```python
from build123d import *

# Parameters (mm, degrees)
SKETCH1_W            = 54.5
SKETCH1_H            = 146
BOSS_EXTRUDE1_DEPTH  = 1.75
SKETCH2_R            = 3.5
SKETCH2_R_2          = 3.795961701
SKETCH2_R_3          = 8
CUT_EXTRUDE1_DEPTH   = 78.939880677
M3_CLEARANCE_HOLE1_D = 3.6
FILLET1_R            = 5


with BuildPart() as part:
    # Sketch1 → Boss-Extrude1 (new body)
    with BuildSketch(Plane(origin=(0, 0, 0), x_dir=(1, 0, 0), z_dir=(0, 1, 0))):
        Rectangle(SKETCH1_W, SKETCH1_H)
    extrude(amount=BOSS_EXTRUDE1_DEPTH)

    # Sketch2 → Cut-Extrude1 (cut, through all)
    with BuildSketch(Plane(origin=(0, 1.75, 0), x_dir=(1, 0, 0), z_dir=(0, 1, 0))):
        with Locations(Location((-19.25, 57, 0), (0, 0, 270))):
            Circle(SKETCH2_R)
        with Locations(Location((-19.25, 0, 0), (0, 0, 270))):
            Circle(SKETCH2_R_2)
        with Locations(Location((-19.25, -57, 0), (0, 0, 90))):
            Circle(SKETCH2_R)
        with Locations(Location((19.25, -57, 0), (0, 0, 270))):
            Circle(SKETCH2_R)
        with Locations(Location((19.25, 0, 0), (0, 0, 90))):
            Circle(SKETCH2_R_2)
        with Locations(Location((19.25, 57, 0), (0, 0, 90))):
            Circle(SKETCH2_R)
        with Locations(Location((0, 0, 0), (0, 0, 270))):
            Circle(SKETCH2_R_3)
        with BuildLine():
            Line((-11.737972568, 9.475230868), (-23.68137085, 21.41862915))
            ThreePointArc((-23.68137085, 21.41862915), (-23.68137085, 23.68137085), (-21.41862915, 23.68137085))
            Line((-21.41862915, 23.68137085), (-9.475230868, 11.737972568))
            ThreePointArc((-9.475230868, 11.737972568), (-9.475230868, 9.475230868), (-11.737972568, 9.475230868))
        make_face()
        with BuildLine():
            Line((11.737972568, 9.475230868), (23.68137085, 21.41862915))
            ThreePointArc((23.68137085, 21.41862915), (23.68137085, 23.68137085), (21.41862915, 23.68137085))
            Line((21.41862915, 23.68137085), (9.475230868, 11.737972568))
            ThreePointArc((9.475230868, 11.737972568), (9.475230868, 9.475230868), (11.737972568, 9.475230868))
        make_face()
        with BuildLine():
            Line((-11.737972568, -9.475230868), (-23.68137085, -21.41862915))
            ThreePointArc((-23.68137085, -21.41862915), (-23.68137085, -23.68137085), (-21.41862915, -23.68137085))
            Line((-21.41862915, -23.68137085), (-9.475230868, -11.737972568))
            ThreePointArc((-9.475230868, -11.737972568), (-9.475230868, -9.475230868), (-11.737972568, -9.475230868))
        make_face()
        with BuildLine():
            Line((11.737972568, -9.475230868), (23.68137085, -21.41862915))
            ThreePointArc((23.68137085, -21.41862915), (23.68137085, -23.68137085), (21.41862915, -23.68137085))
            Line((21.41862915, -23.68137085), (9.475230868, -11.737972568))
            ThreePointArc((9.475230868, -11.737972568), (9.475230868, -9.475230868), (11.737972568, -9.475230868))
        make_face()
        with BuildLine():
            Line((-9.357792216, 68.20993346), (-6.161205405, 68.20993346))
            ThreePointArc((-6.161205405, 68.20993346), (-3.661205405, 65.70993346), (-6.161205405, 63.20993346))
            Line((-6.161205405, 63.20993346), (-9.357792216, 63.20993346))
            ThreePointArc((-9.357792216, 63.20993346), (-11.857792216, 65.70993346), (-9.357792216, 68.20993346))
        make_face()
        with BuildLine():
            Line((-9.357792216, 58.20993346), (-6.161205405, 58.20993346))
            ThreePointArc((-6.161205405, 58.20993346), (-3.661205405, 55.70993346), (-6.161205405, 53.20993346))
            Line((-6.161205405, 53.20993346), (-9.357792216, 53.20993346))
            ThreePointArc((-9.357792216, 53.20993346), (-11.857792216, 55.70993346), (-9.357792216, 58.20993346))
        make_face()
        with BuildLine():
            Line((9.357792216, 58.20993346), (6.161205405, 58.20993346))
            ThreePointArc((6.161205405, 58.20993346), (3.661205405, 55.70993346), (6.161205405, 53.20993346))
            Line((6.161205405, 53.20993346), (9.357792216, 53.20993346))
            ThreePointArc((9.357792216, 53.20993346), (11.857792216, 55.70993346), (9.357792216, 58.20993346))
        make_face()
        with BuildLine():
            Line((-9.357792216, 48.20993346), (-6.161205405, 48.20993346))
            ThreePointArc((-6.161205405, 48.20993346), (-3.661205405, 45.70993346), (-6.161205405, 43.20993346))
            Line((-6.161205405, 43.20993346), (-9.357792216, 43.20993346))
            ThreePointArc((-9.357792216, 43.20993346), (-11.857792216, 45.70993346), (-9.357792216, 48.20993346))
        make_face()
        with BuildLine():
            Line((9.357792216, 48.20993346), (6.161205405, 48.20993346))
            ThreePointArc((6.161205405, 48.20993346), (3.661205405, 45.70993346), (6.161205405, 43.20993346))
            Line((6.161205405, 43.20993346), (9.357792216, 43.20993346))
            ThreePointArc((9.357792216, 43.20993346), (11.857792216, 45.70993346), (9.357792216, 48.20993346))
        make_face()
        with BuildLine():
            Line((-9.357792216, 38.20993346), (-6.161205405, 38.20993346))
            ThreePointArc((-6.161205405, 38.20993346), (-3.661205405, 35.70993346), (-6.161205405, 33.20993346))
            Line((-6.161205405, 33.20993346), (-9.357792216, 33.20993346))
            ThreePointArc((-9.357792216, 33.20993346), (-11.857792216, 35.70993346), (-9.357792216, 38.20993346))
        make_face()
        with BuildLine():
            Line((9.357792216, 68.20993346), (6.161205405, 68.20993346))
            ThreePointArc((6.161205405, 68.20993346), (3.661205405, 65.70993346), (6.161205405, 63.20993346))
            Line((6.161205405, 63.20993346), (9.357792216, 63.20993346))
            ThreePointArc((9.357792216, 63.20993346), (11.857792216, 65.70993346), (9.357792216, 68.20993346))
        make_face()
        with BuildLine():
            Line((9.357792216, 38.20993346), (6.161205405, 38.20993346))
            ThreePointArc((6.161205405, 38.20993346), (3.661205405, 35.70993346), (6.161205405, 33.20993346))
            Line((6.161205405, 33.20993346), (9.357792216, 33.20993346))
            ThreePointArc((9.357792216, 33.20993346), (11.857792216, 35.70993346), (9.357792216, 38.20993346))
        make_face()
        with BuildLine():
            Line((-9.357792216, 28.20993346), (-6.161205405, 28.20993346))
            ThreePointArc((-6.161205405, 28.20993346), (-3.661205405, 25.70993346), (-6.161205405, 23.20993346))
            Line((-6.161205405, 23.20993346), (-9.357792216, 23.20993346))
            ThreePointArc((-9.357792216, 23.20993346), (-11.857792216, 25.70993346), (-9.357792216, 28.20993346))
        make_face()
        with BuildLine():
            Line((9.357792216, 28.20993346), (6.161205405, 28.20993346))
            ThreePointArc((6.161205405, 28.20993346), (3.661205405, 25.70993346), (6.161205405, 23.20993346))
            Line((6.161205405, 23.20993346), (9.357792216, 23.20993346))
            ThreePointArc((9.357792216, 23.20993346), (11.857792216, 25.70993346), (9.357792216, 28.20993346))
        make_face()
        with BuildLine():
            Line((-9.357792216, -68.20993346), (-6.161205405, -68.20993346))
            ThreePointArc((-6.161205405, -68.20993346), (-3.661205405, -65.70993346), (-6.161205405, -63.20993346))
            Line((-6.161205405, -63.20993346), (-9.357792216, -63.20993346))
            ThreePointArc((-9.357792216, -63.20993346), (-11.857792216, -65.70993346), (-9.357792216, -68.20993346))
        make_face()
        with BuildLine():
            Line((-9.357792216, -58.20993346), (-6.161205405, -58.20993346))
            ThreePointArc((-6.161205405, -58.20993346), (-3.661205405, -55.70993346), (-6.161205405, -53.20993346))
            Line((-6.161205405, -53.20993346), (-9.357792216, -53.20993346))
            ThreePointArc((-9.357792216, -53.20993346), (-11.857792216, -55.70993346), (-9.357792216, -58.20993346))
        make_face()
        with BuildLine():
            Line((9.357792216, -58.20993346), (6.161205405, -58.20993346))
            ThreePointArc((6.161205405, -58.20993346), (3.661205405, -55.70993346), (6.161205405, -53.20993346))
            Line((6.161205405, -53.20993346), (9.357792216, -53.20993346))
            ThreePointArc((9.357792216, -53.20993346), (11.857792216, -55.70993346), (9.357792216, -58.20993346))
        make_face()
        with BuildLine():
            Line((-9.357792216, -48.20993346), (-6.161205405, -48.20993346))
            ThreePointArc((-6.161205405, -48.20993346), (-3.661205405, -45.70993346), (-6.161205405, -43.20993346))
            Line((-6.161205405, -43.20993346), (-9.357792216, -43.20993346))
            ThreePointArc((-9.357792216, -43.20993346), (-11.857792216, -45.70993346), (-9.357792216, -48.20993346))
        make_face()
        with BuildLine():
            Line((9.357792216, -48.20993346), (6.161205405, -48.20993346))
            ThreePointArc((6.161205405, -48.20993346), (3.661205405, -45.70993346), (6.161205405, -43.20993346))
            Line((6.161205405, -43.20993346), (9.357792216, -43.20993346))
            ThreePointArc((9.357792216, -43.20993346), (11.857792216, -45.70993346), (9.357792216, -48.20993346))
        make_face()
        with BuildLine():
            Line((-9.357792216, -38.20993346), (-6.161205405, -38.20993346))
            ThreePointArc((-6.161205405, -38.20993346), (-3.661205405, -35.70993346), (-6.161205405, -33.20993346))
            Line((-6.161205405, -33.20993346), (-9.357792216, -33.20993346))
            ThreePointArc((-9.357792216, -33.20993346), (-11.857792216, -35.70993346), (-9.357792216, -38.20993346))
        make_face()
        with BuildLine():
            Line((9.357792216, -68.20993346), (6.161205405, -68.20993346))
            ThreePointArc((6.161205405, -68.20993346), (3.661205405, -65.70993346), (6.161205405, -63.20993346))
            Line((6.161205405, -63.20993346), (9.357792216, -63.20993346))
            ThreePointArc((9.357792216, -63.20993346), (11.857792216, -65.70993346), (9.357792216, -68.20993346))
        make_face()
        with BuildLine():
            Line((9.357792216, -38.20993346), (6.161205405, -38.20993346))
            ThreePointArc((6.161205405, -38.20993346), (3.661205405, -35.70993346), (6.161205405, -33.20993346))
            Line((6.161205405, -33.20993346), (9.357792216, -33.20993346))
            ThreePointArc((9.357792216, -33.20993346), (11.857792216, -35.70993346), (9.357792216, -38.20993346))
        make_face()
        with BuildLine():
            Line((-9.357792216, -28.20993346), (-6.161205405, -28.20993346))
            ThreePointArc((-6.161205405, -28.20993346), (-3.661205405, -25.70993346), (-6.161205405, -23.20993346))
            Line((-6.161205405, -23.20993346), (-9.357792216, -23.20993346))
            ThreePointArc((-9.357792216, -23.20993346), (-11.857792216, -25.70993346), (-9.357792216, -28.20993346))
        make_face()
        with BuildLine():
            Line((9.357792216, -28.20993346), (6.161205405, -28.20993346))
            ThreePointArc((6.161205405, -28.20993346), (3.661205405, -25.70993346), (6.161205405, -23.20993346))
            Line((6.161205405, -23.20993346), (9.357792216, -23.20993346))
            ThreePointArc((9.357792216, -23.20993346), (11.857792216, -25.70993346), (9.357792216, -28.20993346))
        make_face()
    extrude(amount=-CUT_EXTRUDE1_DEPTH, mode=Mode.SUBTRACT)

    # M3 Clearance Hole1 (through all)
    with Locations(Plane(origin=(0, 1.75, 0), x_dir=(1, 0, 0), z_dir=(0, 1, 0))):
        with Locations((-21.25, 67), (21.25, -67), (-21.25, -67), (-21.25, 31), (21.25, 67), (21.25, 31), (21.25, -31), (-21.25, -31), (-15.25, -7.65)):
            Hole(M3_CLEARANCE_HOLE1_D / 2)

    # Fillet1
    fillet1_edges = [part.edges().sort_by_distance(p)[0] for p in [
        (27.25, 0.875, 73),
        (-27.25, 0.875, 73),
        (-27.25, 0.875, -73),
        (27.25, 0.875, -73),
    ]]
    fillet(fillet1_edges, radius=FILLET1_R)


solid = part.part
```
Could you check a few things on this model? Use its own coordinates, in mm. Coordinates: 2 decimals unless noted, no trailing zeros. Order: outer loops, then holes, each group sorted by start corner. A loop starts at its lowest first (then second) coordinate and runs counter-clockwise, first axis right, second up. Notation, with made-up numbers: M 81,-7.75 L 135,-7.75 A26 cw 135,11.25 Z; hole C -6,84.5 d10. An arc over 180 degrees is marked long. Use one line per item in the form item = value. Start each with the question number.
1. Suppose I cut it at B-B on x = 0. Write out the boundary of the cut face in (y, z), then the cut area to 4 significant figures.
2. Suppose I cut it at D-D on y = 1.25. Count the separate pieces of the cut face and the enclosed holes in it, then the cut area to 3 significant figures.
3. Suppose I cut it at C-C on z = 0. Write out the boundary of the cut face in (x, y), then the cut area to 3 significant figures.
4. Suppose I cut it at A-A on z = -31. Write out the boundary of the cut face in (x, y).
5. We'd pull the mould along Z, two halves only. Please class faces 1 (the cylindrical face through (-25.82, 0.89, 71.5)), 2 (the cylindrical face through (3.66, 0.89, -25.76)): +Z half, -Z half, draft (parallel to the pull), parting line (faces both ways), or undercut.
6. Please list where these lines run through material, in increasing order: line 1 (X direction, y = 0.8, z = 0); line 2 (X direction, y = 0.25, z = 59); line 3 (X direction, y = 0.4, z = -31).
Geometry says:
q1.outline = M 0,-73 L 1.75,-73 L 1.75,-8 L 0,-8 Z; M 0,8 L 1.75,8 L 1.75,73 L 0,73 Z
q1.area = 227.5 mm^2
q2.separate_pieces = 1
q2.enclosed_holes = 40
q2.area = 6,440 mm^2
q3.outline = M -27.25,0 L -23.05,0 L -23.05,1.75 L -27.25,1.75 Z; M -15.45,0 L -8,0 L -8,1.75 L -15.45,1.75 Z; M 8,0 L 15.45,0 L 15.45,1.75 L 8,1.75 Z; M 23.05,0 L 27.25,0 L 27.25,1.75 L 23.05,1.75 Z
q3.area = 40.8 mm^2
q4.outline = M -27.25,0 L -23.05,0 L -23.05,1.75 L -27.25,1.75 Z; M -19.45,0 L 19.45,0 L 19.45,1.75 L -19.45,1.75 Z; M 23.05,0 L 27.25,0 L 27.25,1.75 L 23.05,1.75 Z
q5.face_1 = +Z half
q5.face_2 = undercut
q6.line_1 = -27.25 to -23.05, -15.45 to -8, 8 to 15.45, 23.05 to 27.25
q6.line_2 = -27.25 to -22.12, -16.38 to 16.38, 22.12 to 27.25
q6.line_3 = -27.25 to -23.05, -19.45 to 19.45, 23.05 to 27.25
